Autodesk Inventor part; units mm, degrees
ref_plane "XZ Plane" through (0, 0, 0) normal (0, 1, 0) x (-1, 0, 0)
ref_plane "XY Plane" through (0, 0, 0) normal (0, 0, 1) x (1, 0, 0)
sketch "Sketch1" plane through (0, 0, 0) normal (0, 1, 0) x (-1, 0, 0)
  line L0 (-273.05, 263.525) -> (-273.05, -263.525)
  line L1 (-273.05, -263.525) -> (273.05, -263.525)
  line L2 (273.05, -263.525) -> (273.05, 263.525)
  line L3 (273.05, 263.525) -> (-273.05, 263.525)
  line L4 (-273.05, 263.525) -> (273.05, -263.525) construction
  line L5 (-273.05, -263.525) -> (273.05, 263.525) construction
  point P0 (0, 0)
  dimension "baseLength" = 527.05
  dimension "baseWidth" = 546.1
extrude "Extrusion1" add sketch "Sketch1" along normal blind 17.78
sketch "Sketch2" plane through (0, 0, 0) normal (0, -1, 0) x (1, 0, 0)
  line L0 (273.05, 263.525) -> (273.05, -263.525)
  line L1 (273.05, 155.575) -> (222.25, 155.575)
  line L2 (222.25, 155.575) -> (222.25, 53.975)
  line L3 (222.25, 53.975) -> (273.05, 53.975)
  line L4 (273.05, 53.975) -> (273.05, 155.575)
  line L5 (-273.05, 263.525) -> (273.05, 263.525)
  point P0 (0, 0)
  dimension "backToEndOfGearBox" = 107.95
  dimension "backToFrontOfGearBox" = 209.55
  dimension "wdithForGearBox" = 50.8
extrude "Extrusion2" cut sketch "Sketch2" against normal through all
mirror "Mirror1" about plane through (0, 0, 0) normal (1, 0, 0) of "Extrusion2"
sketch "Sketch3" plane through (0, 17.78, 0) normal (0, 1, 0) x (1, 0, 0)
  line L0 (273.05, -225.425) -> (260.35, -225.425)
  line L1 (260.35, -225.425) -> (260.35, -200.025)
  line L2 (260.35, -200.025) -> (273.05, -200.025)
  line L3 (273.05, -200.025) -> (273.05, -225.425)
  line L4 (273.05, -263.525) -> (273.05, -155.575)
  line L5 (-273.05, -263.525) -> (273.05, -263.525)
  point P0 (0, 0)
  dimension "d9" = 25.4
  dimension "d10" = 12.7
  dimension "d11" = 38.1
extrude "Extrusion3" cut sketch "Sketch3" against normal through all
mirror "Mirror2" about plane through (0, 0, 0) normal (1, 0, 0) of "Extrusion3"
sketch "Sketch4" plane through (0, 17.78, 0) normal (0, 1, 0) x (1, 0, 0)
  line L0 (273.05, -53.975) -> (273.05, 263.525)
  line L1 (273.05, 3.175) -> (260.35, 3.175)
  line L2 (260.35, 3.175) -> (260.35, 28.575)
  line L3 (260.35, 28.575) -> (273.05, 28.575)
  line L4 (273.05, 28.575) -> (273.05, 3.175)
  line L5 (-273.05, -263.525) -> (273.05, -263.525)
  point P0 (0, 0)
  dimension "d14" = 25.4
  dimension "d15" = 266.7
  dimension "d16" = 12.7
extrude "Extrusion4" cut sketch "Sketch4" against normal through all
mirror "Mirror3" about plane through (0, 0, 0) normal (1, 0, 0) of "Extrusion4"
sketch "Sketch5" plane through (0, 17.78, 0) normal (0, 1, 0) x (1, 0, 0)
  line L0 (273.05, 231.775) -> (260.35, 231.775)
  line L1 (260.35, 231.775) -> (260.35, 263.525)
  line L2 (260.35, 263.525) -> (273.05, 263.525)
  line L3 (273.05, 263.525) -> (273.05, 231.775)
  line L4 (273.05, 28.575) -> (273.05, 263.525)
  line L5 (273.05, 263.525) -> (-273.05, 263.525)
  point P0 (0, 0)
  dimension "d19" = 12.7
  dimension "d20" = 31.75
extrude "Extrusion5" cut sketch "Sketch5" against normal through all
mirror "Mirror4" about plane through (0, 0, 0) normal (1, 0, 0) of "Extrusion5"
sketch "Sketch8" plane through (0, 17.78, 0) normal (0, 1, 0) x (1, 0, 0)
  line L0 (-76.2, 263.525) -> (76.2, 263.525)
  line L1 (76.2, 263.525) -> (76.2, 174.625)
  line L2 (76.2, 174.625) -> (-76.2, 174.625)
  line L3 (-76.2, 174.625) -> (-76.2, 263.525)
  line L4 (260.35, 263.525) -> (-260.35, 263.525)
  point P0 (0, 0)
  dimension "d23" = 76.2
  dimension "d24" = 76.2
  dimension "d25" = 88.9
extrude "Extrusion6" cut sketch "Sketch8" against normal through all
equation "\"baseLength\" = userBaseLength"
equation "\"baseWidth\" = userBaseWidth"
equation "\"d9\" = lengthOfSpacingForBolt"
equation "\"d10\" = widthOfSpacingForBolt"
equation "\"d11\" = distanceFromBackForEndBolt"
equation "\"d14\" = lengthOfSpacingForBolt"
equation "\"d16\" = widthOfSpacingForBolt"
equation "\"d19\" = widthOfSpacingForBolt"
equation "\"spaceingAlongSides\" = 3.175"
equation "\"distanceFromBackForEndBolt\" = 38.1"
equation "\"widthOfSpacingForBolt\" = 12.7"
equation "\"lengthOfSpacingForBolt\" = 25.4"
equation "\"userBaseLength\" = 527.05"
equation "\"userBaseWidth\" = 546.1"
properties part number "RhinoBottomFloorPlate01" material "Wood (Birch)"
Could you check a few things on this model? Use its own coordinates, in mm. A direction names the side the tool comes from. Give positions to 0.01 mm unless a question says otherwise; leave off trailing zeros. Order: outer loops, then holes, each group sorted by start corner. A loop starts at its lowest first (then second) coordinate and runs counter-clockwise, first axis right, second up. Notation, with made-up numbers: (-27.75, 77.5) -> (8.25, 77.5) arc R19 ccw to (8.25, 112.5) -> close; hole circle Ø7 at (71, 36.5). An arc over 180 degrees is marked (long way). Answer in a Markdown table with one row per item. Add a question column.
Item 1: Imagine slicing it at C-C (z = 85). List the corners of the cut face in (x, y) for me.
Item 2: I'm going to push flat-ended pins straight in: P1, Ø4, axis at x = -267, y = 4.5, coming from the -Z side (3 decimals); P2, Ø9, axis at y = 11, z = -248, coming from the +X side; P3, Ø9, axis at y = 13, z = 218.5, coming from the -X side. Where does each tip first touch, or does it pass through?
Item 3: We'd pull the mould along X, two halves only. Please class faces 1 (the flat face through (247, 9, 53.975)), 2 (the flat face through (-273.05, 9, 177)), 3 (the flat face through (260.35, 9, 213)), 4 (the flat face through (76.2, 9, -220)): pulls with the +X half, pulls with the -X half, needs draft (parallel to the pull), parting line crosses it, or undercut.
Item 4: Please list where these lines run through material, in increasing order: probe 1 along Z at (x, y) = (243.5, 6) (3 decimals); probe 2 along X at (y, z) = (11.75, -240.5); probe 3 along Z at (x, y) = (69, 1) (3 decimals).
Item 5: Imagine slicing it at A-A (z = -221.5). List the corners of the cut face in (x, y) for me.
Item 6: For faces 5 (the flat face through (267, 9, -231.775)), 6 (the flat face through (1, 9, -174.625)), 7 (the flat face through (-260.35, 9, 213)), 8 (the flat face through (-260.35, 9, -248)), which set-ups out of +Z, -Z, +X, -X, +Y, -Y let a thin tool reach every point of the face, with its end or its side?
Item 7: Imagine slicing it at B-B (x = 22). List the corners of the cut face in (y, z) for me (3 decimals), and give its area (3 significant figures).
Result:
| question | item | result |
|---|---|---|
| 1 | outline | (-222.25, 0) -> (222.25, 0) -> (222.25, 17.78) -> (-222.25, 17.78) -> close |
| 2 | P1 | z = -231.775 |
| 2 | P2 | x = 260.35 |
| 2 | P3 | x = -260.35 |
| 3 | face 1 | needs draft |
| 3 | face 2 | pulls with the -X half |
| 3 | face 3 | pulls with the +X half |
| 3 | face 4 | undercut |
| 4 | probe 1 | -263.525 to 53.975, 155.575 to 263.525 |
| 4 | probe 2 | -260.35 to -76.2, 76.2 to 260.35 |
| 4 | probe 3 | -174.625 to 263.525 |
| 5 | outline | (-273.05, 0) -> (-76.2, 0) -> (-76.2, 17.78) -> (-273.05, 17.78) -> close; (76.2, 0) -> (273.05, 0) -> (273.05, 17.78) -> (76.2, 17.78) -> close |
| 6 | face 5 | -Z, +X, +Y, -Y |
| 6 | face 6 | -Z, +Y, -Y |
| 6 | face 7 | -X, +Y, -Y |
| 6 | face 8 | -Z, -X, +Y, -Y |
| 7 | outline | (0, -174.625) -> (17.78, -174.625) -> (17.78, 263.525) -> (0, 263.525) -> close |
| 7 | area | 7,790 mm2 |
